Geometry: final body of the model. Coordinates: model frame, mm. A direction names the side the tool comes from. Coordinates: 2 decimals unless noted, no trailing zeros. Write each loop counter-clockwise with the first axis right and the second up, starting at its lowest first coordinate (ties: lowest second). Pieces come first, ordered by that corner, then holes. Notation, with made-up numbers: M -17.75,29.5 L 14.25,29.5 A30 cw 14.25,54.5 Z; hole C 22,72 d3. An arc over 180 degrees is marked long. Write item = value, one per line. Start each with the question number.
Item 1: Section A-A on z = 14.55. Output: boundary loops of the cut face in (x, y) (3 decimals), plus the area to 3 significant figures.
Item 2: Section B-B on y = -9. Output: boundary loops of the cut face in (x, z), plus the area to 3 significant figures.
Item 3: First-contact query: pin 1 Ø3.5 at (x, z) = (9.5, 34.55) entering from -Y; pin 2 Ø1.5 at (x, y) = (13, -26.56) entering from +Z; pin 3 Ø3 at (x, z) = (13, 38) entering from -Y; pin 4 Ø3 at (x, y) = (6, -14.44) entering from -Z. Flat tips, straight axial feed; report the tip coordinate or a pass-through.
Item 4: Pull-direction query (X, two-part tool) for faces 1 (the cylindrical face through (8.25, -27.55, 45.88)), 2 (the flat face through (9, -16, 49.1)), 3 (the cylindrical face through (2.857, -27.291, 45.881)), 4 (the flat face through (19, -6, 25)); classes: +X half, -X half, draft (parallel to the pull), parting line (faces both ways), or undercut.
Item 5: Reachability of faces 5 (the flat face through (9, -6.35, 25)), 6 (the cylindrical face through (14.6, -17.8, 45.9)) from +Z, -Z, +X, -X, +Y, -Y: full face, straight path, thin tool, end or side. Return the list, or none.
Item 6: Ray query, L1, parallel to Y at x = 9.5, z = 4; L2, parallel to X at y = -15.5, z = 46; L3, parallel to Z at x = 11, y = -10. Return the intervals inside material, ascending. Write a range as [from, to].
Item 7: Section D-D on x = 6. Output: boundary loops of the cut face in (y, z), plus the area to 3 significant figures.
Item 8: Section C-C on y = -17. Output: boundary loops of the cut face in (x, z), plus the area to 3 significant figures.
from build123d import *
from OCP.BRepFilletAPI import BRepFilletAPI_MakeFillet

# Parameters (mm, degrees)
BOSS_EXTRUDE1_DEPTH                            = 19
FILLET1_R                                      = 9.5
F_2_5MM_DOWEL_HOLE1_D                          = 2.5
CIRPATTERN1_COUNT                              = 12
FILLET2_R1                                     = 3
FILLET2_R2                                     = 1.5
F_2_5MM_DOWEL_HOLE2_D                          = 2.5
CSK_FOR_M2_5_FLAT_HEAD_MACHINE_SCREW1_AT_COUNT = 2
CSK_FOR_M2_5_FLAT_HEAD_MACHINE_SCREW1_AT_PITCH = 20


with BuildPart() as part:
    # Sketch16 → Boss-Extrude1 (new body)
    with BuildSketch(Plane(origin=(0, 0, 0), x_dir=(0, 0, -1), z_dir=(1, 0, 0))):
        Polygon((0, 0), (-49.1, 0), (-49.1, -30), (-42.75, -30), (-42.75, -6.35), (-6.35, -6.35), (-6.35, -30), (0, -30), align=None)
    extrude(amount=BOSS_EXTRUDE1_DEPTH)

    # Fillet1
    fillet1_edges = [part.edges().sort_by_distance(p)[0] for p in [
        (19, -30, 3.175),
        (0, -30, 3.175),
        (0, -30, 45.925),
        (19, -30, 45.925),
    ]]
    fillet(fillet1_edges, radius=FILLET1_R - 0.0001)  # a hair under: the kernel refuses the full size

    # Ø2.5mm Dowel Hole1 (through all)
    with Locations(Plane.XY.offset(49.1)):
        with Locations((9.5, -13.5)):
            f_2_5mm_dowel_hole1 = Hole(F_2_5MM_DOWEL_HOLE1_D / 2)

    # CirPattern1: Ø2.5mm Dowel Hole1 ×12 about axis
    cirpattern1_axis = Axis((9.5, -20.5, 0), (0, 0, 1))
    for i in range(1, CIRPATTERN1_COUNT):
        add(f_2_5mm_dowel_hole1.rotate(cirpattern1_axis, i * 360 / CIRPATTERN1_COUNT), mode=Mode.SUBTRACT)

    # Fillet2: one fillet with a radius per group of edges: ONE call of the kernel's fillet builder (fillet() takes one radius for all edges)
    fillet2_edges_1 = [part.edges().sort_by_distance(p)[0] for p in [
        (9.5, 0, 49.1),
        (9.5, 0, 0),
    ]]
    fillet2_edges_2 = [part.edges().sort_by_distance(p)[0] for p in [
        (9.5, -6.35, 42.75),
        (9.5, -6.35, 6.35),
    ]]
    fillet2 = BRepFilletAPI_MakeFillet(part.part.solid().wrapped)
    for e in fillet2_edges_1:
        fillet2.Add(FILLET2_R1, e.wrapped)
    for e in fillet2_edges_2:
        fillet2.Add(FILLET2_R2, e.wrapped)
    add(Compound.cast(fillet2.Shape()), mode=Mode.REPLACE)

    # Ø2.5mm Dowel Hole2 (through all)
    with Locations(Plane.XY.offset(49.1)):
        with Locations((9.5, -20.5)):
            Hole(F_2_5MM_DOWEL_HOLE2_D / 2)

    # Sketch28 → CSK for M2.5 Flat Head Machine Screw1 (revolve, cut)
    with BuildSketch(Plane(origin=(9.5, -6.35, 34.55), x_dir=(0, 0, -1), z_dir=(1, 0, 0))):
        Polygon((0, 0), (0, 6.35), (1.475, 6.35), (1.45, 6.325), (1.45, 1.3), (2.75, 0), align=None)
    csk_for_m2_5_flat_head_machine_screw1 = revolve(axis=Axis((9.5, -12.7, 34.55), (0, 1, 0)), mode=Mode.SUBTRACT)

    # CSK for M2.5 Flat Head Machine Screw1 at: CSK for M2.5 Flat Head Machine Screw1 ×2
    with Locations(*[(0, 0, -i * CSK_FOR_M2_5_FLAT_HEAD_MACHINE_SCREW1_AT_PITCH) for i in range(1, CSK_FOR_M2_5_FLAT_HEAD_MACHINE_SCREW1_AT_COUNT)]):
        add(csk_for_m2_5_flat_head_machine_screw1, mode=Mode.SUBTRACT)


solid = part.part
Responses:
q1.outline = M 0,-6.35 L 6.75,-6.35 L 8.05,-5.05 L 8.05,-0.025 L 8.025,0 L 0,0 Z; M 10.95,-5.05 L 12.25,-6.35 L 19,-6.35 L 19,0 L 10.975,0 L 10.95,-0.025 Z
q1.area = 101 mm²
q2.outline = M 0,0 L 19,0 L 19,6.35 L 0,6.35 Z; M 0,42.75 L 19,42.75 L 19,49.1 L 0,49.1 Z
q2.area = 241 mm²
q3.pin_1 = -5.35
q3.pin_2 = through
q3.pin_3 = -6.35
q3.pin_4 = 0
q4.face_1 = undercut
q4.face_2 = draft
q4.face_3 = -X half
q4.face_4 = +X half
q5.face_5 = +X, -X, -Y
q5.face_6 = +Z, -Z
q6.L1 = [-30, -28.75], [-26.25, -21.75], [-19.25, -14.75], [-12.25, 0]
q6.L2 = [0, 5.34], [6.66, 12.34], [13.66, 19]
q6.L3 = [0, 6.35], [42.75, 49.1]
q7.outline = M -29.33,0 L -27.81,0 L -27.81,6.35 L -29.33,6.35 Z; M -29.33,42.75 L -27.81,42.75 L -27.81,49.1 L -29.33,49.1 Z; M -25.31,0 L -15.69,0 L -15.69,6.35 L -25.31,6.35 Z; M -25.31,42.75 L -15.69,42.75 L -15.69,49.1 L -25.31,49.1 Z; M -13.19,0 L -3,0 A3 ccw 0,3 L 0,46.1 A3 ccw -3,49.1 L -13.19,49.1 L -13.19,42.75 L -7.85,42.75 A1.5 cw -6.35,41.25 L -6.35,7.85 A1.5 cw -7.85,6.35 L -13.19,6.35 Z
q7.area = 537 mm²
q8.outline = M 0,0 L 2.19,0 L 2.19,6.35 L 0,6.35 Z; M 0,42.75 L 2.19,42.75 L 2.19,49.1 L 0,49.1 Z; M 4.69,0 L 14.31,0 L 14.31,6.35 L 4.69,6.35 Z; M 4.69,42.75 L 14.31,42.75 L 14.31,49.1 L 4.69,49.1 Z; M 16.81,0 L 19,0 L 19,6.35 L 16.81,6.35 Z; M 16.81,42.75 L 19,42.75 L 19,49.1 L 16.81,49.1 Z
q8.area = 178 mm²
